from build123d import *

# Parameters (mm, degrees)
SKETCH1_W               = 100.076
SKETCH1_H               = 228.6
BOSS_EXTRUDE1_DEPTH     = 9.525
SKETCH2_W               = 81.026
SKETCH2_H               = 76.2
CUT_EXTRUDE1_DEPTH      = 10.525
SKETCH3_W               = 20.32
SKETCH3_H               = 41.148
SKETCH3_W_2             = 10.9982
SKETCH3_H_2             = 5.08
CUT_EXTRUDE2_DEPTH      = 10.525
SKETCH4_R               = 2.38125
CUT_EXTRUDE3_DEPTH      = 91.551
CUT_EXTRUDE3_DEPTH_BACK = 10.525
SKETCH6_R               = 3.175
CUT_EXTRUDE5_DEPTH      = 10.525
SKETCH5_R               = 2.032
SKETCH5_R_2             = 3.175
CUT_EXTRUDE4_DEPTH      = 1
CUT_EXTRUDE4_DEPTH_BACK = 10.525


with BuildPart() as part:
    # Sketch1 → Boss-Extrude1 (new body)
    with BuildSketch(Plane(origin=(0, 0, 0), x_dir=(1, 0, 0), z_dir=(0, 1, 0))):
        Rectangle(SKETCH1_W, SKETCH1_H)
    extrude(amount=BOSS_EXTRUDE1_DEPTH)

    # Sketch2 → Cut-Extrude1 (cut, through all)
    with BuildSketch(Plane(origin=(0, 9.525, 0), x_dir=(1, 0, 0), z_dir=(0, 1, 0))):
        with Locations((0, -76.2)):
            Rectangle(SKETCH2_W, SKETCH2_H)
    extrude(amount=-CUT_EXTRUDE1_DEPTH, mode=Mode.SUBTRACT)

    # Sketch3 → Cut-Extrude2 (cut, through all)
    with BuildSketch(Plane(origin=(0, 9.525, 0), x_dir=(1, 0, 0), z_dir=(0, 1, 0))):
        with Locations((-30.353, -4.826)):
            Rectangle(SKETCH3_W, SKETCH3_H)
        with Locations((-35.0139, 30.988)):
            Rectangle(SKETCH3_W_2, SKETCH3_H_2)
        with Locations((30.353, -4.826)):
            Rectangle(SKETCH3_W, SKETCH3_H)
        with Locations((35.0139, 30.988)):
            Rectangle(SKETCH3_W_2, SKETCH3_H_2)
    extrude(amount=-CUT_EXTRUDE2_DEPTH, mode=Mode.SUBTRACT)

    # Sketch4 → Cut-Extrude3 (cut, two sides)
    with BuildSketch(Plane(origin=(-40.513, 0, 0), x_dir=(0, 0, -1), z_dir=(1, 0, 0))) as cut_extrude3_sk:
        with Locations((-76.2, 4.7625)):
            Circle(SKETCH4_R)
    extrude(amount=CUT_EXTRUDE3_DEPTH, mode=Mode.SUBTRACT)
    extrude(cut_extrude3_sk.sketch, amount=-CUT_EXTRUDE3_DEPTH_BACK, mode=Mode.SUBTRACT)

    # Sketch6 → Cut-Extrude5 (cut, through all)
    with BuildSketch(Plane(origin=(0, 9.525, 0), x_dir=(1, 0, 0), z_dir=(0, 1, 0))):
        with Locations((0, 39.878)):
            Circle(SKETCH6_R)
    extrude(amount=-CUT_EXTRUDE5_DEPTH, mode=Mode.SUBTRACT)

    # Sketch5 → Cut-Extrude4 (cut, two sides)
    with BuildSketch(Plane(origin=(0, 9.525, 0), x_dir=(1, 0, 0), z_dir=(0, 1, 0))) as cut_extrude4_sk:
        with Locations((-25.273, 19.558)):
            Circle(SKETCH5_R)
        with Locations((-25.273, -29.21)):
            Circle(SKETCH5_R)
        with Locations((25.273, -29.21)):
            Circle(SKETCH5_R)
        with Locations((25.273, 19.558)):
            Circle(SKETCH5_R)
        with Locations((-33.02, 77.978)):
            Circle(SKETCH5_R_2)
        with Locations((33.02, 77.978)):
            Circle(SKETCH5_R_2)
    extrude(amount=CUT_EXTRUDE4_DEPTH, mode=Mode.SUBTRACT)
    extrude(cut_extrude4_sk.sketch, amount=-CUT_EXTRUDE4_DEPTH_BACK, mode=Mode.SUBTRACT)


solid = part.part
CAD build for the part. Positions are in the model's coordinates, mm. A direction names the side the tool comes from. Give positions to 0.01 mm unless a question says otherwise; leave off trailing zeros. Write each loop counter-clockwise with the first axis right and the second up, starting at its lowest first coordinate (ties: lowest second). Pieces come first, ordered by that corner, then holes. Notation, with made-up numbers: (-20.75, 12.25) - (20.25, 12.25) arc R34 ccw to (20.25, 48.25) - close; hole circle Ø8 at (33, -16.75). An arc over 180 degrees is marked (long way). Put each result on its own line as item: value.
(1) Saw through at C-C (z = 29.21). List the corners of the cut face in (x, y) (3 decimals), then the cut area to 3 significant figures.
Working result:
outline: (-50.038, 0) - (-27.305, 0) - (-27.305, 9.525) - (-50.038, 9.525) - close; (-23.241, 0) - (23.241, 0) - (23.241, 9.525) - (-23.241, 9.525) - close; (27.305, 0) - (50.038, 0) - (50.038, 9.525) - (27.305, 9.525) - close
area: 876 mm^2
(2) Saw through at A-A (z = 76.2). List the corners of the cut face in (x, y) (3 decimals), then the cut area to 3 significant figures.
Working result:
outline: (-50.038, 0) - (-40.513, 0) - (-40.513, 2.381) - (-50.038, 2.381) - close; (-50.038, 7.144) - (-40.513, 7.144) - (-40.513, 9.525) - (-50.038, 9.525) - close; (40.513, 0) - (50.038, 0) - (50.038, 2.381) - (40.513, 2.381) - close; (40.513, 7.144) - (50.038, 7.144) - (50.038, 9.525) - (40.513, 9.525) - close
area: 90.7 mm^2
(3) Pull direction Z, two halves, no side cores. Call faces 1 (the flat face through (-30, 5, -15.748)), 2 (the flat face through (-1, 9.525, -27)), 3 (the flat face through (45, 5, 114.3)), 4 (the flat face through (30, 5, -15.748)): released by +Z, released by -Z, zero draft, split by the parting line, or undercut.
Working result:
face 1: undercut
face 2: zero draft
face 3: released by +Z
face 4: undercut
(4) Wall check: L1, parallel to X at y = 2.25, z = 15; L2, parallel to Z at x = -25, y = 8.5; L3, parallel to X at y = 2.5, z = -77.5. Give the ranges that are in metal, low to high.
Working result:
L1: -50.04 to -40.51, -20.19 to 20.19, 40.51 to 50.04
L2: -114.3 to -21.57, -17.54 to -15.75, 25.4 to 27.2, 31.22 to 38.1
L3: -50.04 to -36.16, -29.88 to 29.88, 36.16 to 50.04
(5) Saw through at D-D (x = 0). List the corners of the cut face in (y, z) (3 decimals), then the cut area to 3 significant figures.
Working result:
outline: (0, -114.3) - (9.525, -114.3) - (9.525, -43.053) - (0, -43.053) - close; (0, -36.703) - (9.525, -36.703) - (9.525, 38.1) - (0, 38.1) - close
area: 1,390 mm^2
(6) Drop flat-ended pins along their axis: pin 1 Ø6 at (x, z) = (37, 82.5) entering from +Y; pin 2 Ø5 at (x, y) = (33.5, 6) entering from +Z. Give the stop position or say it passes through.
Working result:
pin 1: through
pin 2: z = 38.1
(7) Saw through at B-B (x = -33.02). List the corners of the cut face in (y, z) (3 decimals), then the cut area to 3 significant figures.
Working result:
outline: (0, -114.3) - (9.525, -114.3) - (9.525, -81.153) - (0, -81.153) - close; (0, -74.803) - (9.525, -74.803) - (9.525, -33.528) - (0, -33.528) - close; (0, -28.448) - (9.525, -28.448) - (9.525, -15.748) - (0, -15.748) - close; (0, 25.4) - (9.525, 25.4) - (9.525, 38.1) - (0, 38.1) - close
area: 951 mm^2
(8) Tool access for faces 5 (the flat face through (-40.513, 2, 77)), 6 (the flat face through (-1, 0, -27)), 7 (the flat face through (29.515, 5, -31)): list every direction of +Z, -Z, +X, -X, +Y, -Y with a clear straight run to the whole face (end or side of a thin tool).
Working result:
face 5: +Z, +Y, -Y
face 6: +Z, -Z, +X, -X, -Y
face 7: +Y, -Y
